```python
from build123d import *

# Parameters (mm, degrees)
BOSS_EXTRUDE1_DEPTH = 46.45
FILLET1_R           = 10
FILLET2_R           = 10
SHELL1_T            = -1.2
BOSS_EXTRUDE2_START = 10
SKETCH2_R           = 1.5
BOSS_EXTRUDE2_DEPTH = 2
CUT_EXTRUDE1_DEPTH  = 1.2
SKETCH4_W           = 3.252453774
SKETCH4_H           = 29.408591544
BOSS_EXTRUDE3_DEPTH = 11
FILLET3_R           = 10
CUT_EXTRUDE2_DEPTH  = 3.252453774


with BuildPart() as part:
    # Sketch1 → Boss-Extrude1 (new body)
    with BuildSketch(Plane.XY):
        with BuildLine():
            Line((-7.6, 131.988), (-72.288, 131.988))
            Line((-72.288, 131.988), (-72.288, -8))
            Line((-72.288, -8), (-15.6, -8))
            ThreePointArc((-15.6, -8), (-9.943145751, -5.656854249), (-7.6, 0))
            Line((-7.6, 0), (-7.6, 131.988))
        make_face()
    extrude(amount=BOSS_EXTRUDE1_DEPTH)

    # Fillet1
    fillet1_edges = [part.edges().sort_by_distance(p)[0] for p in [
        (-72.288, 131.988, 23.225),
    ]]
    fillet(fillet1_edges, radius=FILLET1_R)

    # Fillet2
    fillet2_edges = [part.edges().sort_by_distance(p)[0] for p in [
        (-72.288, 56.994, 46.45),
        (-69.359067812, 129.059067812, 46.45),
        (-34.944, 131.988, 46.45),
    ]]
    fillet(fillet2_edges, radius=FILLET2_R)

    # Shell1
    shell1_openings = [part.faces().sort_by_distance(p)[0] for p in [
        (-7.6, 65.770031668, 23.151264626),
        (-43.729452835, -8, 23.052515396),
        (-9.943145751, -5.656854249, 23.225),
        (-39.918891594, 61.936645467, 0),
    ]]
    offset(amount=SHELL1_T, openings=shell1_openings, kind=Kind.INTERSECTION)

    # Sketch2 → Boss-Extrude2 (add)
    # profile 1 of 2: a face of its own
    with BuildSketch(Plane.XY.offset(BOSS_EXTRUDE2_START)):
        with BuildLine():
            Line((-76.288, 120.488), (-72.288, 120.488))
            Line((-72.288, 120.488), (-72.288, 113.488))
            Line((-72.288, 113.488), (-76.288, 113.488))
            ThreePointArc((-76.288, 113.488), (-79.788, 116.988), (-76.288, 120.488))
        make_face()
        with Locations((-76.288, 116.988)):
            Circle(SKETCH2_R, mode=Mode.SUBTRACT)
    # profile 2 of 2: a face of its own
    with BuildSketch(Plane.XY.offset(BOSS_EXTRUDE2_START)):
        with BuildLine():
            Line((-76.288, 30.488), (-72.288, 30.488))
            Line((-72.288, 30.488), (-72.288, 23.488))
            Line((-72.288, 23.488), (-76.288, 23.488))
            ThreePointArc((-76.288, 23.488), (-79.788, 26.988), (-76.288, 30.488))
        make_face()
        with Locations((-76.288, 26.988)):
            Circle(SKETCH2_R, mode=Mode.SUBTRACT)
    extrude(amount=BOSS_EXTRUDE2_DEPTH)

    # Sketch3 → Cut-Extrude1 (cut)
    with BuildSketch(Plane.ZY.offset(72.288)):
        with BuildLine():
            Line((0, 12), (13.45, 12))
            ThreePointArc((13.45, 12), (33.45, -8), (13.45, -28))
            Line((13.45, -28), (0, -28))
            ThreePointArc((0, -28), (-20, -8), (0, 12))
        make_face()
    extrude(amount=-CUT_EXTRUDE1_DEPTH, mode=Mode.SUBTRACT)

    # Sketch4 → Boss-Extrude3 (add)
    with BuildSketch(Plane.ZY.offset(72.288)):
        with Locations((34.823773113, 61.979262262)):
            Rectangle(SKETCH4_W, SKETCH4_H)
    extrude(amount=BOSS_EXTRUDE3_DEPTH)

    # Fillet3
    fillet3_edges = [part.edges().sort_by_distance(p)[0] for p in [
        (-83.288, 76.683558034, 34.823773113),
        (-83.288, 47.27496649, 34.823773113),
    ]]
    fillet(fillet3_edges, radius=FILLET3_R)

    # Sketch5 → Cut-Extrude2 (cut)
    with BuildSketch(Plane.XY.offset(36.45)):
        with BuildLine():
            Line((-80.288, 66.683558034), (-80.288, 57.27496649))
            ThreePointArc((-80.288, 57.27496649), (-78.90048608, 53.091666357), (-75.288, 50.566762558))
            Line((-75.288, 50.566762558), (-75.288, 73.391761966))
            ThreePointArc((-75.288, 73.391761966), (-78.90048608, 70.866858166), (-80.288, 66.683558034))
        make_face()
    extrude(amount=-CUT_EXTRUDE2_DEPTH, mode=Mode.SUBTRACT)


solid = part.part
```
Read the model definition and answer for the solid it produces. Units are mm, in the model's axes. A direction names the side the tool comes from. Give positions to 0.01 mm unless a question says otherwise; leave off trailing zeros. Order: outer loops, then holes, each group sorted by start corner. A loop starts at its lowest first (then second) coordinate and runs counter-clockwise, first axis right, second up. Notation, with made-up numbers: (-30.5, 66) -> (-19.5, 66) arc R29 ccw to (-19.5, 94) -> close; hole circle Ø2 at (-26, -19.5). An arc over 180 degrees is marked (long way). One line per item, written item: value. Start each with the question number.
(1) The part is cut by section A-A (y = 61). Determine the outline of the cut face in (x, z), and give its area (3 significant figures).
(2) The part is cut by section B-B (z = 7.5). Determine the outline of the cut face in (x, y), and give its area (3 significant figures).
(3) A tool of negligible diameter and unlimited length cuts with its end or side. For faces 1 (the flat face through (-80.288, 62, 35)), 2 (the flat face through (-74, 117, 12)), 3 (the flat face through (-75, 62, 33.198)), 4 (the cylindrical face through (-68.44, 128.28, 18.48)), from which of +Z, -Z, +X, -X, +Y, -Y can it reach the whole face along a straight path? Write none if from no direction.
(4) The part is cut by section C-C (x = -51). Determine the outline of the cut face in (y, z), and give its area (3 significant figures).
(5) For a pull along Y with two mould halves and no side action, classify faces 5 (the cylindrical face through (-80.281, 50.127, 34.847)), 6 (the cylindrical face through (-69.28, 129.14, 18.48)), 7 (the cylindrical face through (-79.787, 26.911, 10.986)), 8 (the cylindrical face through (-68.44, 56.08, 42.74)) as released by +Y, released by -Y, zero draft, split by the parting line, or undercut.
(6) Flat-ended cylindrical pins translate along their axes: P1, Ø0.6, axis at x = -74, z = 11, coming from the +Y side; P2, Ø5.5, axis at x = -77.5, y = 118.5, coming from the +Z side; P3, Ø8, axis at y = 51.5, z = 25.5, coming from the +X side. Find the tip coordinate at first contact, or state that the pin passes through.
(7) Straight lines are drawn through the part: L1, parallel to Z at x = -39, y = 13; L2, parallel to Y at x = -30, z = 16.5; L3, parallel to X at y = 94, z = 21. For each, find the intervals that lie inside material, in ascending order.
Taken from the geometry:
1. outline: (-83.29, 33.2) -> (-80.29, 33.2) -> (-80.29, 36.45) -> (-83.29, 36.45) -> close; (-75.29, 33.2) -> (-72.29, 33.2) -> (-72.29, 0) -> (-71.09, 0) -> (-71.09, 36.45) arc R8.8 cw to (-62.29, 45.25) -> (-7.6, 45.25) -> (-7.6, 46.45) -> (-62.29, 46.45) arc R10 ccw to (-72.29, 36.45) -> (-75.29, 36.45) -> close
1. area: 147 mm^2
2. outline: (-72.29, 12) -> (-71.09, 12) -> (-71.09, 121.99) arc R8.8 cw to (-62.29, 130.79) -> (-7.6, 130.79) -> (-7.6, 131.99) -> (-62.29, 131.99) arc R10 ccw to (-72.29, 121.99) -> close
2. area: 215 mm^2
3. face 1: +Z, -Z
3. face 2: +Z, -X, +Y, -Y
3. face 3: -Z, -X, +Y, -Y
3. face 4: -Z, +X, -Y
4. outline: (-8, 45.25) -> (121.99, 45.25) arc R8.8 cw to (130.79, 36.45) -> (130.79, 0) -> (131.99, 0) -> (131.99, 36.45) arc R10 ccw to (121.99, 46.45) -> (-8, 46.45) -> close
4. area: 217 mm^2
5. face 5: released by -Y
5. face 6: released by +Y
5. face 7: undercut
5. face 8: zero draft
6. P1: y = 120.49
6. P2: z = 12
6. P3: x = -71.09
7. L1: 45.25 to 46.45
7. L2: 130.79 to 131.99
7. L3: -72.29 to -71.09
